For this review, take the finished solid that the model builds, in its own axes (mm). Coordinates: 2 decimals unless noted, no trailing zeros. Write each loop counter-clockwise with the first axis right and the second up, starting at its lowest first coordinate (ties: lowest second). Pieces come first, ordered by that corner, then holes. Notation, with made-up numbers: M 2,7.5 L 11,7.5 A16 cw 11,11.5 Z; hole C 44,52.25 d1. An arc over 180 degrees is marked long. One line per question, with ' | ' between items.
Autodesk Inventor part; units mm, degrees
ref_plane "YZ Plane" through (0, 0, 0) normal (1, 0, 0) x (0, 1, 0)
ref_plane "XZ Plane" through (0, 0, 0) normal (0, 1, 0) x (-1, 0, 0)
ref_plane "XY Plane" through (0, 0, 0) normal (0, 0, 1) x (1, 0, 0)
sketch "Sketch1" plane through (0, 0, 0) normal (0, 0, 1) x (1, 0, 0)
  line L0 (-6, 60) -> (-6, -60)
  line L1 (-6, -64) -> (-6, -66.5)
  line L2 (-6, -66.5) -> (-2, -66.5)
  line L3 (-2, -66.5) -> (-2, -64)
  line L4 (-2, -64) -> (2, -64)
  line L5 (2, -64) -> (2, -66.5)
  line L6 (2, -66.5) -> (6, -66.5)
  line L7 (6, -66.5) -> (6, -64)
  line L8 (6, -60) -> (6, 60)
  line L9 (0, 63.1461) -> (0, -63.1461) construction
  line L10 (-16.7969, 0) -> (16.7969, 0) construction
  arc A0 (6, 60) -> (-6, 60) centre (0, 70.3923) ccw
  circle A1 centre (-2.0706, 78.1197) radius 1.7678
  line L11 (-2.0706, 90.8634) -> (-2.0706, 65.376) construction
  line L12 (-3.3097, 78.1197) -> (-0.8314, 78.1197) construction
  line L13 (-3.3206, 79.3697) -> (-0.8206, 79.3697) construction
  line L14 (-0.8206, 79.3697) -> (-0.8206, 76.8697) construction
  line L15 (-0.8206, 76.8697) -> (-3.3206, 76.8697) construction
  line L16 (-3.3206, 76.8697) -> (-3.3206, 79.3697) construction
  circle A2 centre (0, 70.3923) radius 8 construction
  line L17 (10, -64) -> (10, -60)
  line L18 (10, -60) -> (6, -60)
  line L19 (-10, -64) -> (-10, -60)
  line L20 (-10, -60) -> (-6, -60)
  line L21 (-10, -64) -> (-6, -64)
  line L22 (6, -64) -> (10, -64)
  line L23 (0, 70.3923) -> (-4.1411, 85.8471) construction
  circle A3 centre (-5.6569, 76.0492) radius 1.7678
  circle A4 centre (-7.7274, 72.4629) radius 1.7678
  circle A5 centre (-7.7274, 68.3218) radius 1.7678
  circle A6 centre (-5.6569, 64.7355) radius 1.7678
  circle A7 centre (-2.0706, 62.6649) radius 1.7678
  circle A8 centre (2.0706, 62.6649) radius 1.7678
  circle A9 centre (5.6569, 64.7355) radius 1.7678
  circle A10 centre (7.7274, 68.3218) radius 1.7678
  circle A11 centre (7.7274, 72.4629) radius 1.7678
  circle A12 centre (5.6569, 76.0492) radius 1.7678
  circle A13 centre (2.0706, 78.1197) radius 1.7678
  line L24 (-4.2764, 70.3923) -> (4.2764, 70.3923) construction
  line L25 (-4, 71.6423) -> (-1.25, 71.6423) construction
  line L26 (-1.25, 71.6423) -> (-1.25, 74.3923) construction
  line L27 (-1.25, 74.3923) -> (1.25, 74.3923) construction
  line L28 (1.25, 74.3923) -> (1.25, 71.6423) construction
  line L29 (1.25, 71.6423) -> (4, 71.6423) construction
  line L30 (4, 71.6423) -> (4, 69.1423) construction
  line L31 (4, 69.1423) -> (1.25, 69.1423) construction
  line L32 (1.25, 69.1423) -> (1.25, 66.3923) construction
  line L33 (1.25, 66.3923) -> (-1.25, 66.3923) construction
  line L34 (-1.25, 66.3923) -> (-1.25, 69.1423) construction
  line L35 (-1.25, 69.1423) -> (-4, 69.1423) construction
  line L36 (-4, 69.1423) -> (-4, 71.6423) construction
  circle A14 centre (0, 70.3923) radius 4.1908
  circle A15 centre (0, 70.3923) radius 6 construction
  point P0 (0, 0)
  point P1 (0, 0)
  point P2 (-5.1993, 77.7567)
  point P3 (-8.1849, 74.1704)
  point P4 (-8.9774, 69.5718)
  point P5 (-7.3644, 65.193)
  point P6 (-3.7781, 62.2074)
  point P7 (0.8206, 61.4149)
  point P8 (5.1993, 63.0279)
  point P9 (8.1849, 66.6142)
  point P10 (8.9774, 71.2129)
  point P11 (7.3644, 75.5916)
  point P12 (3.7781, 78.5772)
  dimension "d9" = 3.5355
  dimension "d10" = 16
  dimension "d0" = 4
  dimension "d2" = 4
  dimension "d7" = 2.5
  dimension "d8" = 2.5
  dimension "d11" = 24
  dimension "d14" = 4
  dimension "d16" = 4
  dimension "d17" = 12
  dimension "d18" = 20
  dimension "d19" = 2.5
  dimension "d20" = 120
  dimension "d21" = 15
  dimension "d24" = 360
  dimension "d28" = 2.5
  dimension "d29" = 2.5
  dimension "d30" = 8
  dimension "d31" = 8
  dimension "d32" = 12
extrude "Extrusion1" add sketch "Sketch1" along normal mid plane 2.5
properties part number "pitahaya1"
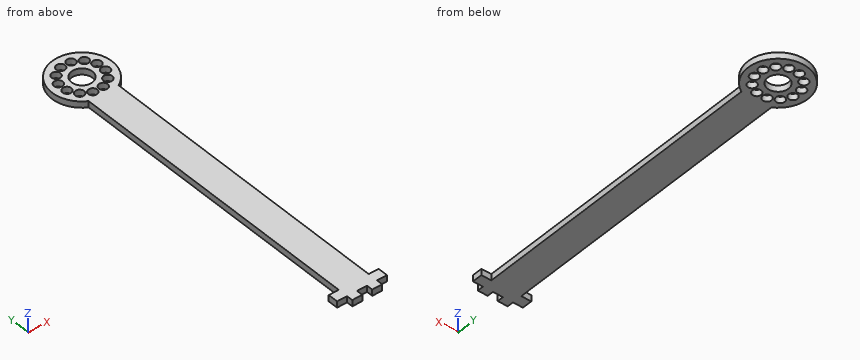
1. Clearance check with flat-ended pins moving along their axes: P1, Ø1.2, axis at y = -65, z = 0, coming from the +X side; P2, Ø0.8, axis at x = 7.5, z = 0.5, coming from the -Y side; P3, Ø11, axis at x = 0, y = 70.39, coming from the -Z side; P4, Ø1.2, axis at y = 16.5, z = -0.5, coming from the -X side. State where each tip first meets the part, or that it passes through.
Computed values:
P1: stops at x = 6 | P2: stops at y = -64 | P3: stops at z = -1.25 | P4: stops at x = -6
2. Take a section at B-B on y = 33. State the section outline as (x, z) points.
Computed values:
outline: M -6,-1.25 L 6,-1.25 L 6,1.25 L -6,1.25 Z
3. For line 1 along Y through (x, z) = (-1, 0.35); line 2 along X through (y, z) = (64.5, -0.9); line 3 along Y through (x, z) = (0.5, 0.9), list the stretches that pass through material, from the lowest coordinate up.
Computed values:
line 1: y = -64 to 61.26, 64.07 to 66.32, 74.46 to 76.71, 79.53 to 82.35 | line 2: x = -10.45 to -7.41, -3.9 to 3.9, 7.41 to 10.45 | line 3: y = -64 to 61.85, 63.48 to 66.23, 74.55 to 77.31, 78.93 to 82.38
4. Take a section at A-A on z = 0.4. Give the number of separate pieces and of enclosed holes in the cut face, plus the area to 3 significant figures.
Computed values:
separate pieces: 1 | enclosed holes: 13 | area: 1,810 mm2
